Input: part model. Units: mm. Frame: model coordinates. A direction names the side the tool comes from. Round coordinates to 2 decimals unless told otherwise and drop trailing zeros. Order: outer loops, then holes, each group sorted by start corner. A loop starts at its lowest first (then second) coordinate and runs counter-clockwise, first axis right, second up. Notation, with made-up numbers: (27.5, 42) -> (55.5, 42) arc R24 ccw to (55.5, 55) -> close; hole circle Ø4 at (-4, 74). An arc over 180 degrees is marked (long way). Use a Markdown table: item, result.
from build123d import *

# Parameters (mm, degrees)
F0_W     = 31.75
F0_H     = 44.45
F1_DEPTH = 5.842
F2_R     = 6.35
F4_DEPTH = 38.1


with BuildPart() as f1:
    # F0 (on Top) → F1 (new body)
    with BuildSketch(Plane.XY):
        Rectangle(F0_W, F0_H)
    extrude(amount=F1_DEPTH)

    # F2
    f2_edges = [f1.edges().sort_by_distance(p)[0] for p in [
        (15.875, 22.225, 2.921),
        (-15.875, 22.225, 2.921),
        (-15.875, -22.225, 2.921),
        (15.875, -22.225, 2.921),
    ]]
    fillet(f2_edges, radius=F2_R)

    # F3 (on face) → F4 (cut)
    with BuildSketch(Plane.XZ.offset(22.225)):
        Polygon((5.08, 2.54), (0, 2.54), (-5.08, 2.54), (-3.175, 0), (3.175, 0), align=None)
    extrude(amount=-F4_DEPTH, mode=Mode.SUBTRACT)


solid = f1.part
1) Cut plane D-D on x = 13. Return loops of the section in (y, z).
Answer key:
| item | result |
|---|---|
| outline | (-21.19, 0) -> (21.19, 0) -> (21.19, 5.84) -> (-21.19, 5.84) -> close |
2) Cut plane C-C on x = -12. Return loops of the section in (y, z).
Answer key:
| item | result |
|---|---|
| outline | (-21.72, 0) -> (21.72, 0) -> (21.72, 5.84) -> (-21.72, 5.84) -> close |
3) Ray query, probe 1 along X at (y, z) = (-11, 0.85) (1 decimal); probe 2 along X at (y, z) = (7.5, 0.6) (3 decimals); probe 3 along Z at (x, y) = (1.5, 13). Return the intervals inside material, ascending.
Answer key:
| item | result |
|---|---|
| probe 1 | x = -15.9 to -3.8, 3.8 to 15.9 |
| probe 2 | x = -15.875 to -3.625, 3.625 to 15.875 |
| probe 3 | z = 2.54 to 5.84 |
4) Cut plane B-B on z = 3. Return loops of the section in (x, y) (3 decimals), and give its area (3 significant figures).
Answer key:
| item | result |
|---|---|
| outline | (-15.875, -15.875) arc R6.35 ccw to (-9.525, -22.225) -> (9.525, -22.225) arc R6.35 ccw to (15.875, -15.875) -> (15.875, 15.875) arc R6.35 ccw to (9.525, 22.225) -> (-9.525, 22.225) arc R6.35 ccw to (-15.875, 15.875) -> close |
| area | 1,380 mm^2 |
5) Draft query along Z for faces 1 (the face through (-4.14, -3.44, 1.29)), 2 (the face through (-14.06, 20.32, 2.96)), 3 (the face through (4.11, -3.44, 1.25)), 4 (the face through (0, 0, 5.842)). Return one class per face: released by +Z, released by -Z, zero draft, split by the parting line, or undercut.
Answer key:
| item | result |
|---|---|
| face 1 | undercut |
| face 2 | zero draft |
| face 3 | undercut |
| face 4 | released by +Z |
6) Cut plane A-A on y = -6. Return loops of the section in (x, z) (3 decimals).
Answer key:
| item | result |
|---|---|
| outline | (-15.875, 0) -> (-3.175, 0) -> (-5.08, 2.54) -> (5.08, 2.54) -> (3.175, 0) -> (15.875, 0) -> (15.875, 5.842) -> (-15.875, 5.842) -> close |
7) Set-up query: faces 5 (the face through (0, 15.875, 1)), 6 (the face through (-15.875, 0, 3)). Return all of +Z, -Z, +X, -X, +Y, -Y with unobstructed straight access to the full face (end or side cutting, diameter ignored); none if empty.
Answer key:
| item | result |
|---|---|
| face 5 | -Y |
| face 6 | +Z, -Z, -X, +Y, -Y |
8) Contact query for flat-ended pins moving along their axis: P1, Ø2, axis at x = 0, z = 1, coming from the -Y side (3 decimals); P2, Ø5, axis at x = -1, y = -9, coming from the -Z side. Output: stop coordinate, or through.
Answer key:
| item | result |
|---|---|
| P1 | stops at y = 15.875 |
| P2 | stops at z = 0 |
